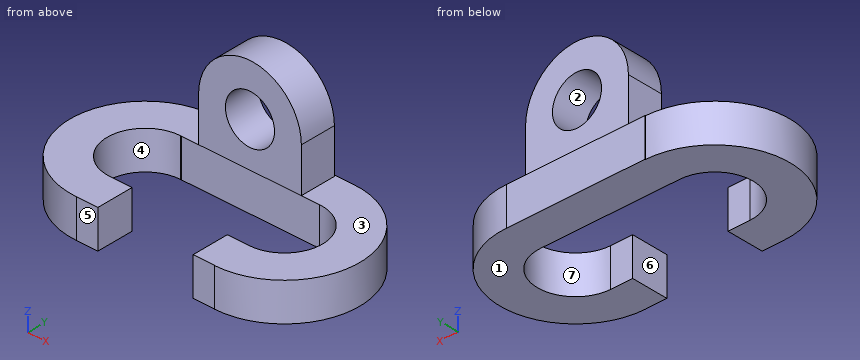
```python
from build123d import *

# Parameters (mm, degrees)
F1_DEPTH = 12.7
F2_R     = 8.183106
F3_DEPTH = 11.938


with BuildPart() as f1:
    # F0 (on Top) → F1 (new body)
    with BuildSketch(Plane.XY):
        with BuildLine():
            ThreePointArc((-23.2029, -12.7), (-35.9029, 0), (-23.2029, 12.7))
            Line((-23.2029, 12.7), (-23.2029, 25.040741))
            ThreePointArc((-23.2029, 25.040741), (-48.24355, -0.067309), (-23.068282, -25.040379))
            Line((-23.068282, -25.040379), (-15.875, -25.040379))
            Line((-15.875, -25.040379), (-15.875, -12.7))
            Line((-15.875, -12.7), (-23.2029, -12.7))
        make_face()
        with BuildLine():
            Line((-22.774086, 12.692759), (23.2029, 12.7))
            Line((23.2029, 12.7), (22.993142, 25.1211))
            Line((22.993142, 25.1211), (-23.2029, 25.204616))
            Line((-23.2029, 25.204616), (-23.2029, 25.040741))
            Line((-23.2029, 25.040741), (-23.2029, 12.7))
            ThreePointArc((-23.2029, 12.7), (-22.988463, 12.69819), (-22.774086, 12.692759))
        make_face()
        with BuildLine():
            ThreePointArc((23.2029, 12.7), (35.9029, 0), (23.2029, -12.7))
            Line((23.2029, -12.7), (15.875, -12.7))
            Line((15.875, -12.7), (15.875, -25.040379))
            Line((15.875, -25.040379), (23.068282, -25.040379))
            Line((23.068282, -25.040379), (23.067396, -25.12161))
            ThreePointArc((23.067396, -25.12161), (48.324848, 0.037128), (22.993142, 25.1211))
            Line((22.993142, 25.1211), (23.2029, 12.7))
        make_face()
    extrude(amount=F1_DEPTH)

    # F2 (on face) → F3 (join)
    with BuildSketch(Plane(origin=(-0.002, 12.696345, 0), x_dir=(1, 0.000158, 0), z_dir=(0.000158, -1, 0))):
        with BuildLine():
            Line((17.135601, 12.7), (17.135601, 27.470101))
            ThreePointArc((17.135601, 27.470101), (0, 44.605702), (-17.135601, 27.470101))
            Line((-17.135601, 27.470101), (-17.135601, 12.7))
            Line((-17.135601, 12.7), (17.135601, 12.7))
        make_face()
        with Locations((0, 27.470101)):
            Circle(F2_R, mode=Mode.SUBTRACT)
    extrude(amount=-F3_DEPTH)


solid = f1.part
```
Here's how the part is built. I have some questions about the finished solid (model axes, mm). Face numbers are marked on the shaded views. A direction names the side the tool comes from. Round coordinates to 2 decimals unless told otherwise and drop trailing zeros. Loops run counter-clockwise (first coordinate to the right, second up) from the corner with the lowest first, then second, coordinate; pieces in that order, holes last.
1. Suppose I cut it at D-D, the plane z = 42.5. Please give me the cut outline in (x, y), and give its area (3 significant figures).
Answers:
outline: (-8.23, 12.7) - (8.23, 12.7) - (8.23, 24.64) - (-8.23, 24.63) - close
area: 196 mm2
2. If I drill on probe 1 along Z at (x, y) = (-27, 23); probe 2 along Y at (x, z) = (10, 20); probe 3 along X at (y, z) = (18, 13), over which ranges is the centre line in solid material (lowest first)?
Answers:
probe 1: z = 0 to 12.7
probe 2: y = 12.7 to 24.64
probe 3: x = -17.14 to 17.13
3. Thinking about a two-plate mould opening in Z: for the marked faces 1, 2, 3 and 4, which applies, released by +Z, released by -Z, zero draft, split by the parting line, or undercut?
Answers:
face 1: released by -Z
face 2: undercut
face 3: released by +Z
face 4: zero draft
4. Suppose I cut it at C-C, the plane z = 16. Please give me the cut outline in (x, y), and give its area (3 significant figures).
Answers:
outline: (-17.14, 12.69) - (17.13, 12.7) - (17.13, 24.64) - (-17.14, 24.63) - close
area: 409 mm2
5. Suppose I cut it at B-B, the plane z = 34. Please give me the cut outline in (x, y).
Answers:
outline: (-15.85, 24.63) - (-15.84, 12.69) - (-4.93, 12.7) - (-4.94, 24.63) - close; (4.93, 12.7) - (15.84, 12.7) - (15.84, 24.64) - (4.93, 24.64) - close
6. Will these pins go through, and if not, where does the flat tip stop? pin 1 (3 mm diameter, centred on x = 20.5, z = 18, fed in from -Y); pin 2 (21.5 mm diameter, centred on x = 0, z = 27.47, fed in from -Y); pin 3 (3.5 mm diameter, centred on y = 18, z = 23.5, fed in from +X); pin 4 (3.5 mm diameter, centred on x = -18.5, z = 8.5, fed in from -Y).
Answers:
pin 1: passes through
pin 2: stops at y = 12.69
pin 3: stops at x = 17.13
pin 4: stops at y = -25.04
7. For the marked faces 5, 6 and 7, which set-ups out of +Z, -Z, +X, -X, +Y, -Y let a thin tool reach every point of the face, with its end or its side?
Answers:
face 5: +Z, -Z, -X, -Y
face 6: +Z, -Z, -Y
face 7: +Z, -Z
8. Suppose I cut it at A-A, the plane y = 0. Please give me the cut outline in (x, z).
Answers:
outline: (-48.24, 0) - (-35.9, 0) - (-35.9, 12.7) - (-48.24, 12.7) - close; (35.9, 0) - (48.32, 0) - (48.32, 12.7) - (35.9, 12.7) - close
